Model file for the job. Use its own axes, mm. Face numbers are marked on the shaded views. A direction names the side the tool comes from. Round coordinates to 2 decimals unless told otherwise and drop trailing zeros. Order: outer loops, then holes, each group sorted by start corner. A loop starts at its lowest first (then second) coordinate and runs counter-clockwise, first axis right, second up. Notation, with made-up numbers: (-8, 70) -> (45, 70) arc R14 ccw to (45, 85) -> close; hole circle Ø7 at (74, 9.5). An arc over 180 degrees is marked (long way). Put each result on its own line as item: value. Start each with the question number.
Q1. Cut at C-C, the plane z = 12.75. List the corners of the cut face in (x, y), and give its area (3 significant figures).
Q2. 3-axis set-ups, long thin cutter, end or side, ignore diameter. For the marked faces 1, 2 and 3: which of +Z, -Z, +X, -X, +Y, -Y reach the whole face in a straight line?
Q3. Pull direction X, two halves, no side cores. Call the marked faces 4, 5, 6 and 7: released by +X, released by -X, zero draft, split by the parting line, or undercut.
Q4. Cut at B-B, the plane y = 28.5. List the corners of the cut face in (x, z), and give its area (3 significant figures).
Q5. Flat gauge pins, fed straight in: P1, Ø7, axis at x = 28.75, z = 0, coming from the +Y side; P2, Ø3, axis at x = 26, y = 25.5, coming from the +Z side; P3, Ø2, axis at x = 29, z = 10, coming from the -Y side. Where does each tip first touch, or does it go through?
Q6. Cut at D-D, the plane x = 18.75. List the corners of the cut face in (y, z).
Q7. Probe L1, parallel to X at y = 24.5, z = -13; L2, parallel to Z at x = 46.5, y = 26; L3, parallel to X at y = 25.25, z = 10.5. List the from-to ranges inside material, lowest first.
Q8. Cut at A-A, the plane x = 49. List the corners of the cut face in (y, z).
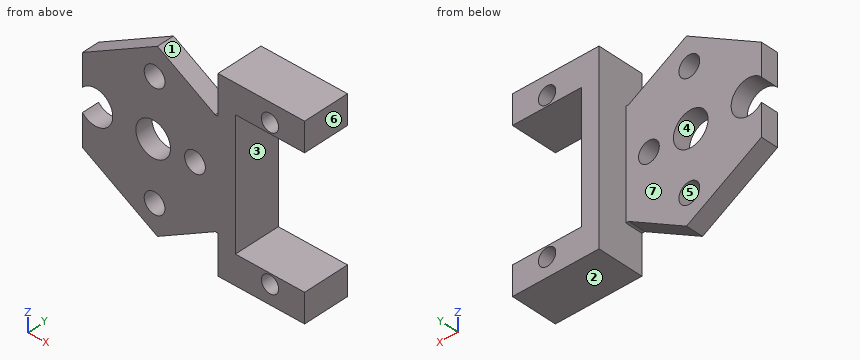
from build123d import *

# Parameters (mm, degrees)
SKETCH180_R     = 1.5
PAD127016_DEPTH = 5
SKETCH178_R     = 1.8
SKETCH178_R_2   = 1.5
SKETCH178_R_3   = 3
PAD127015_DEPTH = 3


with BuildPart() as pad127016:
    # Sketch180 → Pad127016 (new body)
    with BuildSketch(Plane.XZ.offset(-27)):
        Polygon((40, -9.220944), (40, 9.220944), (40, 16), (55, 16), (55, 11), (43, 11), (43, -11), (55, -11), (55, -16), (40, -16), align=None)
        with Locations((49, 12.75)):
            Circle(SKETCH180_R, mode=Mode.SUBTRACT)
        with Locations((49, -12.75)):
            Circle(SKETCH180_R, mode=Mode.SUBTRACT)
    extrude(amount=-PAD127016_DEPTH)


with BuildPart() as brakemount:
    # Sketch178 → Pad127015 (new body)
    with BuildSketch(Plane.XZ.offset(-27)):
        with BuildLine():
            Line((29.490381, 15), (16.5, 7.5))
            Line((16.5, 1.984313), (16.5, 7.5))
            ThreePointArc((16.5, -1.984313), (21.75, 0), (16.5, 1.984313))
            Line((16.5, -1.984313), (16.5, -7.5))
            Line((16.5, -7.5), (29.490381, -15))
            Line((29.490381, -15), (39.5, -9.220944))
            Line((39.5, -9.220944), (40, -9.220944))
            Line((40, -16), (40, -9.220944))
            Line((55, -16), (40, -16))
            Line((55, -11), (55, -16))
            Line((55, -11), (43, -11))
            Line((43, -11), (43, 11))
            Line((43, 11), (55, 11))
            Line((55, 11), (55, 16))
            Line((55, 16), (40, 16))
            Line((40, 16), (40, 9.220944))
            Line((39.5, 9.220944), (40, 9.220944))
            Line((29.490381, 15), (39.5, 9.220944))
        make_face()
        with Locations((29, 10)):
            Circle(SKETCH178_R, mode=Mode.SUBTRACT)
        with Locations((36, 0)):
            Circle(SKETCH178_R, mode=Mode.SUBTRACT)
        with Locations((29, -10)):
            Circle(SKETCH178_R, mode=Mode.SUBTRACT)
        with Locations((49, 12.75)):
            Circle(SKETCH178_R_2, mode=Mode.SUBTRACT)
        with Locations((49, -12.75)):
            Circle(SKETCH178_R_2, mode=Mode.SUBTRACT)
        with Locations((28.75, 0)):
            Circle(SKETCH178_R_3, mode=Mode.SUBTRACT)
    extrude(amount=PAD127015_DEPTH)

    # Fusion004020019: union Pad127016
    add(pad127016.part)


solid = brakemount.part
Ans:
1. outline: (25.59, 24) -> (33.39, 24) -> (33.39, 27) -> (25.59, 27) -> close; (40, 24) -> (47.5, 24) -> (47.5, 32) -> (40, 32) -> close; (50.5, 24) -> (55, 24) -> (55, 32) -> (50.5, 32) -> close
1. area: 119 mm^2
2. face 1: +Z, +Y, -Y
2. face 2: -Z, +X, -X, +Y, -Y
2. face 3: +X, +Y, -Y
3. face 4: undercut
3. face 5: undercut
3. face 6: released by +X
3. face 7: zero draft
4. outline: (40, -16) -> (55, -16) -> (55, -11) -> (43, -11) -> (43, 11) -> (55, 11) -> (55, 16) -> (40, 16) -> close; hole circle Ø3 at (49, -12.75); hole circle Ø3 at (49, 12.75)
4. area: 202 mm^2
5. P1: stops at y = 27
5. P2: stops at z = 13.85
5. P3: passes through
6. outline: (24, -8.8) -> (27, -8.8) -> (27, -3) -> (24, -3) -> close; (24, 3) -> (27, 3) -> (27, 8.8) -> (24, 8.8) -> close
7. L1: x = 26.03 to 32.95, 40 to 47.52, 50.48 to 55
7. L2: z = -16 to -11, 11 to 16
7. L3: x = 21.7 to 27.27, 30.73 to 37.28, 40 to 43
8. outline: (24, -16) -> (32, -16) -> (32, -14.25) -> (24, -14.25) -> close; (24, -11.25) -> (32, -11.25) -> (32, -11) -> (24, -11) -> close; (24, 11) -> (32, 11) -> (32, 11.25) -> (24, 11.25) -> close; (24, 14.25) -> (32, 14.25) -> (32, 16) -> (24, 16) -> close
